Verification items for the finished model (mm, model axes). A direction names the side the tool comes from. Give positions to 0.01 mm unless a question says otherwise; leave off trailing zeros. Loops run counter-clockwise (first coordinate to the right, second up) from the corner with the lowest first, then second, coordinate; pieces in that order, holes last. Notation, with made-up numbers: (34.5, 12.25) - (51.5, 12.25) arc R16 cw to (51.5, 35.25) - close; hole circle Ø5 at (-30.5, 46.5). An arc over 180 degrees is marked (long way). Put each result on its own line as item: value. Start each with the question number.
```python
from build123d import *

# Parameters (mm, degrees)
BOSS_EXTRUDE1_DEPTH   = 6.35
FILLET1_R             = 1.5875
M4X0_7_TAPPED_HOLE1_D = 3.3


with BuildPart() as part:
    # Sketch3 → Boss-Extrude1 (new, symmetric)
    with BuildSketch(Plane.XY):
        Polygon((3.175, 19.05), (0, 19.05), (0, 0), (19.05, 0), (19.05, 3.175), (3.175, 3.175), align=None)
    extrude(amount=BOSS_EXTRUDE1_DEPTH, both=True)

    # Fillet1
    fillet1_edges = [part.edges().sort_by_distance(p)[0] for p in [
        (3.175, 3.175, 0),
        (19.05, 3.175, 0),
        (3.175, 19.05, 0),
    ]]
    fillet(fillet1_edges, radius=FILLET1_R)

    # M4x0.7 Tapped Hole1 (through all)
    with Locations(Plane(origin=(3.175, 0, 0), x_dir=(0, 0, -1), z_dir=(1, 0, 0))):
        with Locations((0, 11.1125)):
            Hole(M4X0_7_TAPPED_HOLE1_D / 2)


solid = part.part
```
1) Depth check by flat-ended pin: P1, Ø5, axis at x = 9.5, z = 2.5, coming from the +Y side (3 decimals); P2, Ø6.5, axis at y = 13.5, z = 2, coming from the +X side (3 decimals); P3, Ø1.5, axis at x = 4.5, z = 4.5, coming from the +Y side. Enter the tip coordinate at first touch or a pass-through.
2) Scan lines: line 1 along Y through (x, z) = (1.2, 0); line 2 along X through (y, z) = (14, 4.5) (3 decimals). Record each from-to range of solid material in increasing order. Write a range as from..to.
3) Set-up check for faces 1 (the face through (11, 3.175, 0)), 2 (the face through (0, 9.7, -1.3)): record each of +Z, -Z, +X, -X, +Y, -Y from which the full face is reachable in a straight line by a thin tool's end or side.
4) Section check C-C, the plane x = 7.75. Enter the section's corners in (y, z) (3 decimals), plus the area to 3 significant figures.
5) Draft check along Y on faces 3 (the face through (9, 0, 0)), 4 (the face through (1.57, 12.75, -0.21)), 5 (the face through (3, 6, 6.35)), 6 (the face through (1, 19.05, 0)). Enter one of: pulls with the +Y half, pulls with the -Y half, needs draft (parallel to the pull), parting line crosses it, or undercut.
Results are:
1. P1: stops at y = 3.175
1. P2: stops at x = 3.175
1. P3: stops at y = 3.54
2. line 1: y = 0..9.46, 12.76..19.05
2. line 2: x = 0..3.175
3. face 1: +Z, -Z, +X, +Y
3. face 2: +Z, -Z, -X, +Y, -Y
4. outline: (0, -6.35) - (3.175, -6.35) - (3.175, 6.35) - (0, 6.35) - close
4. area: 40.3 mm2
5. face 3: pulls with the -Y half
5. face 4: undercut
5. face 5: needs draft
5. face 6: pulls with the +Y half
